Autodesk Inventor part; units mm, degrees
ref_plane "YZ Plane" through (0, 0, 0) normal (1, 0, 0) x (0, 1, 0)
ref_plane "XZ Plane" through (0, 0, 0) normal (0, 1, 0) x (-1, 0, 0)
ref_plane "XY Plane" through (0, 0, 0) normal (0, 0, 1) x (1, 0, 0)
sketch "スケッチ1" plane through (0, 0, 0) normal (0, 1, 0) x (-1, 0, 0)
  line L0 (13.25, -2) -> (-13.25, -2)
  line L1 (-13.25, -2) -> (-13.25, 2)
  line L2 (13.25, 2) -> (13.25, -2)
  line L3 (13.25, 2) -> (4, 16.5)
  line L4 (4, 16.5) -> (0, 16.5)
  line L5 (0, 16.5) -> (-13.25, 2)
  line L6 (9.25, 3.5) -> (-9.25, 3.5)
  line L7 (9.25, 3.5) -> (9.25, -2)
  line L8 (-9.25, 3.5) -> (-9.25, -2)
  point P0 (0, 0)
  point P1 (13.25, 0)
  point P2 (0, -2)
  point P3 (2, 16.5)
  dimension "d1" = 4
  dimension "d2" = 4
  dimension "d3" = 16.5
  dimension "d19" = 3.5
  dimension "d32" = 4
  dimension "d33" = 26.5
  dimension "d34" = 4
  dimension "d36" = 4
  dimension "d37" = 2
extrude "押し出し1" add sketch "スケッチ1" along normal mid plane 4 contours L0 L7 L6 L8 L1 L5 L4 L3 L2
sketch "スケッチ3" plane through (-4, 2, 16.5) normal (0, 0, 1) x (1, 0, 0)
  line L0 (0, 0) -> (4, 0)
  line L1 (0, -4) -> (0, 0)
  point P0 (4, -2)
  point P1 (2, -2)
  point P2 (0, -2)
  point P3 (2, 0)
hole "穴1" at (-2, 0, 16.5) direction (0, 0, -1) diameter 2 end through all
sketch "スケッチ4" plane through (13.25, -2, -2) normal (1, 0, 0) x (0, 0, -1)
  line L0 (0, 4) -> (0, 0)
  line L1 (-4, 0) -> (-4, 4)
  line L2 (0, 0) -> (-4, 0)
  circle A0 centre (-2, 2) radius 1.2
  line L3 (-4, 4) -> (0, 4)
  arc A1 (-4, 0) -> (-4, 4) centre (-2, 2) ccw
  circle A2 centre (-0.9929, 3.7444) radius 0.8142
  circle A3 centre (-0.9929, 0.2556) radius 0.8142
  line L4 (-0.9929, 3.7444) -> (-2, 2) construction
  line L5 (-2, 2) -> (-0.9929, 0.2556) construction
  line L6 (-0.9929, 1.0699) -> (-0.9929, 2.9301) construction
  line L7 (0, 2.2089) -> (-0.9929, 3.7444) construction
  point P0 (-2, 2)
  point P1 (-1.4, 3.0392)
  point P2 (-1.4, 0.9608)
  point P3 (-0.2199, 0)
  point P4 (-0.2199, 4)
  point P5 (-0.5858, 4.4495)
  point P6 (-0.5858, -0.4495)
  dimension "d22" = 1.6284
  dimension "d20" = 2.4
  dimension "d21" = 120
  dimension "d23" = 1.8603
extrude "押し出し3" add sketch "スケッチ4" against normal up to surface (4 mm away)
extrude "押し出し4" cut sketch "スケッチ4" against normal up to surface (4 mm away) contours A1 L0 | L0 L2 A3 A0 A2 L3 | L3 A2 A1 | A1 A3 L2 | A0 picked at (-0.1339, 4.0556) picked at (-0.1339, -0.0556)
mirror "ミラー1" about plane through (0, 0, 0) normal (1, 0, 0) of "押し出し3", "押し出し4"
sketch "スケッチ5" plane through (0, 2, 0) normal (0, 1, 0) x (1, 0, 0)
  line L0 (-13.25, -2) -> (-4, -16.5)
  line L1 (-4, -16.5) -> (0, -16.5)
  line L2 (0, -16.5) -> (13.25, -2)
  line L3 (9.25, -3.5) -> (-9.25, -3.5)
  line L4 (-2.9036, -14.5) -> (-8.6449, -5.5)
  line L5 (7.3425, -5.5) -> (-0.8817, -14.5)
  line L6 (-0.8817, -14.5) -> (-2.9036, -14.5)
  line L7 (-8.6449, -5.5) -> (7.3425, -5.5)
  point P0 (0, 0)
  dimension "d38" = 2
  dimension "d40" = 2
  dimension "d41" = 2
extrude "押し出し5" cut sketch "スケッチ5" against normal through all
fillet "フィレット4" radius 1.5 2 edges at (-8.6449, 0, 5.5) (7.3425, 0, 5.5)
fillet "フィレット5" radius 2 6 edges at (9.25, 0, 3.5) (-9.25, 0, 3.5) (-11.25, 2, 2) (11.25, 2, 2) (11.25, -2, 2) (-11.25, -2, 2)
equation "\"d34\" = d32"
equation "\"d36\" = d1"
equation "\"d40\" = d38"
equation "\"d41\" = d38"
properties part number "GearBase" material "ABS プラスチック"
Part model, mm, in its own coordinate system. A direction names the side the tool comes from. Round coordinates to 2 decimals unless told otherwise and drop trailing zeros. Write each loop counter-clockwise with the first axis right and the second up, starting at its lowest first coordinate (ties: lowest second). Pieces come first, ordered by that corner, then holes. Notation, with made-up numbers: (-15, -12) -> (15, -12) arc R34 cw to (15, 27) -> close; hole circle Ø2 at (11.25, -38). An arc over 180 degrees is marked (long way). Return JSON: item names as keys, results as strings. Group by question number.
Q1. Pin check, flat tips, straight feed: pin 1 (1 mm diameter, centred on x = 7, z = 1.5, fed in from -Y); pin 2 (4 mm diameter, centred on x = 6, z = 10.5, fed in from +Y); pin 3 (2 mm diameter, centred on y = 2, z = 7, fed in from -X); pin 4 (1 mm diameter, centred on x = -2, y = 1, fed in from -Z). Stop position of each tip, or through.
Q2. Saw through at B-B on z = 0. Write the cut outline in (x, y).
Q3. Saw through at A-A on y = 0. Write the cut outline in (x, z).
Q4. Mould opens along X. For faces 1 (the flat face through (2.124, 0.028, 11.211)), 2 (the flat face through (13.25, 0, 1.4)), 3 (the flat face through (-8.69, -0.03, 9.15)), 4 (the flat face through (0, -2, 5)) say: pulls with the +X half, pulls with the -X half, needs draft (parallel to the pull), parting line crosses it, or undercut.
Q5. Saw through at D-D on z = 6.25. Write the cut outline in (x, y).
Q6. Saw through at C-C on x = -2. Write the cut outline in (y, z), plus the area to 3 significant figures.
Q7. Which spindle directions (+Z, -Z, +X, -X, +Y, -Y) get a long thin tool onto all of the face, cutting with end or side? Do faces 5 (the cylindrical face through (-7.235, -0.028, 6.299)), 6 (the flat face through (-3, -1, 16.5)), 7 (the flat face through (0, 0, 3.5)). Say none if no direction does.
Q8. Probe L1, parallel to Y at x = -11.4, z = 0; L2, parallel to Y at x = -2, z = 4.8; L3, parallel to Y at x = 1.75, z = 12.5. List the from-to ranges inside material, lowest first. Write a range as [from, to].
Answer:
{
 "1": {"pin 1": "through", "pin 2": "y = 2", "pin 3": "x = -10.7", "pin 4": "z = 3.5"},
 "2": {"outline": "(-13.25, -2.83) -> (-9.25, -2.83) -> (-9.25, -1.2) -> (-13.25, -1.2) -> close; (-13.25, 1.2) -> (-9.25, 1.2) -> (-9.25, 2.83) -> (-13.25, 2.83) -> close; (9.25, -2.83) -> (13.25, -2.83) -> (13.25, -1.2) -> (9.25, -1.2) -> close; (9.25, 1.2) -> (13.25, 1.2) -> (13.25, 2.83) -> (9.25, 2.83) -> close"},
 "3": {"outline": "(-13.25, 1.2) -> (-9.25, 1.2) -> (-9.25, 1.5) arc R2 cw to (-7.25, 3.5) -> (-3, 3.5) -> (-3, 5.5) -> (-5.91, 5.5) arc R1.5 cw to (-7.17, 7.81) -> (-3, 14.35) -> (-3, 16.5) -> (-4, 16.5) -> (-13.25, 2) -> close; (-1, 3.5) -> (7.25, 3.5) arc R2 cw to (9.25, 1.5) -> (9.25, 1.2) -> (13.25, 1.2) -> (13.25, 2) -> (0, 16.5) -> (-1, 16.5) -> (-1, 14.5) -> (-0.88, 14.5) -> (5.05, 8.01) arc R1.5 cw to (3.94, 5.5) -> (-1, 5.5) -> close"},
 "4": {"face 1": "undercut", "face 2": "pulls with the +X half", "face 3": "pulls with the -X half", "face 4": "needs draft"},
 "5": {"outline": "(-10.54, -2) -> (-7.21, -2) -> (-7.21, 2) -> (-10.54, 2) -> close; (5.24, -2) -> (9.37, -2) -> (9.37, 2) -> (5.24, 2) -> close"},
 "6": {"outline": "(-2, 3.5) -> (-1, 3.5) -> (-1, 5.5) -> (-2, 5.5) -> close; (-2, 14.5) -> (-1, 14.5) -> (-1, 16.5) -> (-2, 16.5) -> close; (1, 3.5) -> (2, 3.5) -> (2, 5.5) -> (1, 5.5) -> close; (1, 14.5) -> (2, 14.5) -> (2, 16.5) -> (1, 16.5) -> close", "area": "8.00 mm2"},
 "7": {"face 5": "+Y, -Y", "face 6": "+Z, +X, -X, +Y, -Y", "face 7": "-Z, +Y, -Y"},
 "8": {"L1": "[-2.83, -1.2], [1.2, 2.83]", "L2": "[-2, -1], [1, 2]", "L3": "[-2, 2]"}
}
